Read the model definition and answer for the solid it produces. Units are mm, in the model's axes. Face numbers are marked on the shaded views. A direction names the side the tool comes from. Round coordinates to 2 decimals unless told otherwise and drop trailing zeros. Loops run counter-clockwise (first coordinate to the right, second up) from the corner with the lowest first, then second, coordinate; pieces in that order, holes last. Notation, with made-up numbers: M 63.25,-21 L 116.25,-21 A17 cw 116.25,7 Z; hole C 31,9 d10. An arc over 180 degrees is marked long. Write each question's results on one line, items separated by ' | '.
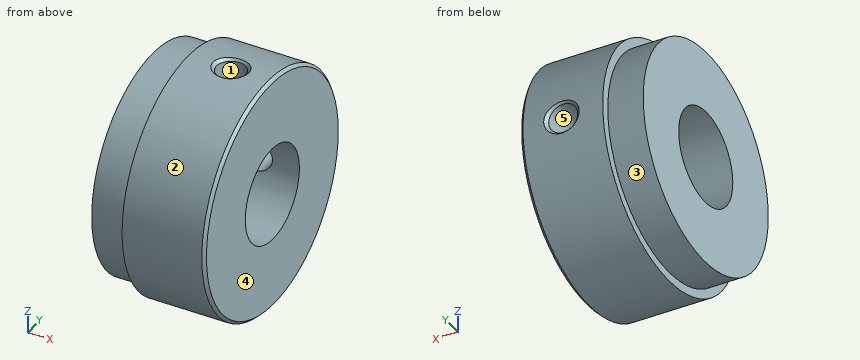
```python
from build123d import *


with BuildPart() as part:
    # Sketch1 → Revolve1 (revolve)
    with BuildSketch(Plane.XY, mode=Mode.PRIVATE) as revolve1_sk:
        Polygon((0, 4), (10, 4), (10, 9.75), (9.75, 10), (3, 10), (3, 9.25), (0, 9.25), align=None)
    revolve(revolve1_sk.sketch.rotate(Axis((10, 0, 0), (-1, 0, 0)), 270), axis=Axis((10, 0, 0), (-1, 0, 0)))

    # Sketch2 → Cut-Revolve1 (revolve, cut)
    with BuildSketch(Plane(origin=(6.5, 0, 0), x_dir=(0, 0, -1), z_dir=(1, 0, 0)), mode=Mode.PRIVATE) as cut_revolve1_sk:
        Polygon((0, 10), (1.5, 10), (1.2295, 9.7295), (1.2295, 0), (0, 0), align=None)
    revolve(cut_revolve1_sk.sketch.rotate(Axis((6.5, 0, 0), (0, 1, 0)), 180), axis=Axis((6.5, 0, 0), (0, 1, 0)), mode=Mode.SUBTRACT)

    # Sketch3 → Cut-Revolve2 (revolve, cut)
    with BuildSketch(Plane(origin=(6.5, 0, 0), x_dir=(0, 0, -1), z_dir=(1, 0, 0)), mode=Mode.PRIVATE) as cut_revolve2_sk:
        Polygon((-10, 0), (-10, 1.5), (-9.7295, 1.2295), (0, 1.2295), (0, 0), align=None)
    revolve(cut_revolve2_sk.sketch.rotate(Axis((6.5, 0, 0), (0, 0, 1)), 180), axis=Axis((6.5, 0, 0), (0, 0, 1)), mode=Mode.SUBTRACT)


solid = part.part
```
1. Find section C-C, the plane x = 6.5. Give the vertices of the cut face in (y, z).
Completed:
outline: M -1.4,9.9 A10 ccw long 9.9,-1.4 L 9.73,-1.23 L 3.81,-1.23 A4 cw long -1.23,3.81 L -1.23,9.73 Z; M 1.23,3.81 A4 cw 3.81,1.23 L 9.73,1.23 L 9.9,1.4 A10 ccw 1.4,9.9 L 1.23,9.73 Z
2. Which of the six approach directions +Z, -Z, +X, -X, +Y, -Y give full straight-line access (tool end or side, diameter ignored) to the marked faces 1 and 2?
Completed:
face 1: +Z | face 2: +X, -X
3. Given P1, Ø6, axis at x = 6.5, z = -4, coming from the +Y side; P2, Ø5, axis at x = 8.5, z = -4.5, coming from the +Y side; P3, Ø1, axis at x = 8, z = 3, coming from the -Y side, each flat-ended and moving along its own axis, determine where each tip first touches the part or whether it passes through.
Completed:
P1: stops at y = 9.94 | P2: stops at y = 9.8 | P3: stops at y = -9.68
4. Find the intervals of material crossed by L1, parallel to Y at x = 0.75, z = 0; L2, parallel to X at y = 7.4, z = 0; L3, parallel to Y at x = 7, z = 7, in increasing order.
Completed:
L1: y = -9.25 to -4, 4 to 9.25 | L2: x = 0 to 5.27, 7.73 to 10 | L3: y = -7.14 to -1.12, 1.12 to 7.14
5. Determine the mould class of the marked faces 3, 4 and 5 for opening direction X: released by +X, released by -X, zero draft, split by the parting line, or undercut.
Completed:
face 3: zero draft | face 4: released by +X | face 5: undercut
6. Find section A-A, the plane z = 0. Give the vertices of the cut face in (x, y), then the cut area to 3 significant figures.
Completed:
outline: M 0,-9.25 L 3,-9.25 L 3,-10 L 9.75,-10 L 10,-9.75 L 10,-4 L 0,-4 Z; M 0,4 L 5.27,4 L 5.27,9.73 L 5,10 L 3,10 L 3,9.25 L 0,9.25 Z; M 7.73,4 L 10,4 L 10,9.75 L 9.75,10 L 8,10 L 7.73,9.73 Z | area: 101 mm2
7. Find section D-D, the plane x = 3.5. Give the vertices of the cut face in (y, z), then the cut area to 3 significant figures.
Completed:
outline: C 0,0 d20; hole C 0,0 d8 | area: 264 mm2
